from build123d import *

# Parameters (mm, degrees)
SKETCH1_W            = 76
SKETCH1_H            = 16
BOSS_EXTRUDE1_DEPTH  = 1.5
SKETCH2_W            = 6
SKETCH2_H            = 6
BOSS_EXTRUDE2_DEPTH  = 4
SKETCH3_R            = 1.75
BOSS_EXTRUDE3_DEPTH  = 1.5
SKETCH7_W            = 6
SKETCH7_H            = 6
BOSS_EXTRUDE4_DEPTH  = 4
SKETCH9_R            = 1.75
BOSS_EXTRUDE5_DEPTH  = 1.5
SKETCH11_W           = 6
SKETCH11_H           = 6
BOSS_EXTRUDE6_DEPTH  = 4
SKETCH13_R           = 1.75
BOSS_EXTRUDE7_DEPTH  = 1.5
SKETCH15_W           = 6
SKETCH15_H           = 6
BOSS_EXTRUDE8_DEPTH  = 4
SKETCH17_R           = 1.75
BOSS_EXTRUDE9_DEPTH  = 1.5
SKETCH19_W           = 6
SKETCH19_H           = 6
BOSS_EXTRUDE10_DEPTH = 4
SKETCH21_R           = 1.75
BOSS_EXTRUDE11_DEPTH = 1.5
SKETCH23_R           = 1.5
BOSS_EXTRUDE12_DEPTH = 7
FILLET1_R            = 1
SKETCH24_W           = 18
SKETCH24_H           = 9
BOSS_EXTRUDE13_DEPTH = 5
M3_CLEARANCE_HOLE2_D = 3.4


with BuildPart() as part:
    # Sketch1 → Boss-Extrude1 (new body)
    with BuildSketch(Plane.XY):
        with Locations((38, 8)):
            Rectangle(SKETCH1_W, SKETCH1_H)
    extrude(amount=BOSS_EXTRUDE1_DEPTH)

    # Sketch2 → Boss-Extrude2 (add)
    with BuildSketch(Plane.XY.offset(1.5)):
        with Locations((6, 5)):
            Rectangle(SKETCH2_W, SKETCH2_H)
    extrude(amount=BOSS_EXTRUDE2_DEPTH)

    # Sketch3 → Boss-Extrude3 (add)
    with BuildSketch(Plane.XY.offset(5.5)):
        with Locations(Location((6.17, 5, 0), (0, 0, 180))):
            Circle(SKETCH3_R)
    extrude(amount=BOSS_EXTRUDE3_DEPTH)

    # Sketch7 → Boss-Extrude4 (add)
    with BuildSketch(Plane(origin=(16.242371321, -0.520498802, 1.5), x_dir=(1, 0, 0), z_dir=(0, 0, 1))):
        with Locations((7.477628679, 5.520498802)):
            Rectangle(SKETCH7_W, SKETCH7_H)
    extrude(amount=BOSS_EXTRUDE4_DEPTH)

    # Sketch9 → Boss-Extrude5 (add)
    with BuildSketch(Plane(origin=(16.242371321, -0.520498802, 5.5), x_dir=(1, 0, 0), z_dir=(0, 0, 1))):
        with Locations(Location((7.477628679, 5.520498802, 0), (0, 0, 180))):
            Circle(SKETCH9_R)
    extrude(amount=BOSS_EXTRUDE5_DEPTH)

    # Sketch11 → Boss-Extrude6 (add)
    with BuildSketch(Plane(origin=(28.595266875, 2.580968484, 1.5), x_dir=(1, 0, 0), z_dir=(0, 0, 1))):
        with Locations((7.724733125, 2.419031516)):
            Rectangle(SKETCH11_W, SKETCH11_H)
    extrude(amount=BOSS_EXTRUDE6_DEPTH)

    # Sketch13 → Boss-Extrude7 (add)
    with BuildSketch(Plane(origin=(28.595266875, 2.580968484, 5.5), x_dir=(1, 0, 0), z_dir=(0, 0, 1))):
        with Locations(Location((7.724733125, 2.419031516, 0), (0, 0, 180))):
            Circle(SKETCH13_R)
    extrude(amount=BOSS_EXTRUDE7_DEPTH)

    # Sketch15 → Boss-Extrude8 (add)
    with BuildSketch(Plane(origin=(42.206058337, 2.089594669, 1.5), x_dir=(1, 0, 0), z_dir=(0, 0, 1))):
        with Locations((9.813941663, 2.910405331)):
            Rectangle(SKETCH15_W, SKETCH15_H)
    extrude(amount=BOSS_EXTRUDE8_DEPTH)

    # Sketch17 → Boss-Extrude9 (add)
    with BuildSketch(Plane(origin=(42.206058337, 2.089594669, 5.5), x_dir=(1, 0, 0), z_dir=(0, 0, 1))):
        with Locations(Location((9.813941663, 2.910405331, 0), (0, 0, 180))):
            Circle(SKETCH17_R)
    extrude(amount=BOSS_EXTRUDE9_DEPTH)

    # Sketch19 → Boss-Extrude10 (add)
    with BuildSketch(Plane(origin=(52.604179533, 1.086479777, 1.5), x_dir=(1, 0, 0), z_dir=(0, 0, 1))):
        with Locations((17.295820467, 3.913520223)):
            Rectangle(SKETCH19_W, SKETCH19_H)
    extrude(amount=BOSS_EXTRUDE10_DEPTH)

    # Sketch21 → Boss-Extrude11 (add)
    with BuildSketch(Plane(origin=(52.604179533, 1.086479777, 5.5), x_dir=(1, 0, 0), z_dir=(0, 0, 1))):
        with Locations(Location((17.295820467, 3.913520223, 0), (0, 0, 180))):
            Circle(SKETCH21_R)
    extrude(amount=BOSS_EXTRUDE11_DEPTH)

    # Sketch23 → Boss-Extrude12 (add)
    with BuildSketch(Plane.XY.offset(1.5)):
        with Locations(Location((6.17, 10.5, 0), (0, 0, 180))):
            Circle(SKETCH23_R)
    extrude(amount=BOSS_EXTRUDE12_DEPTH)

    # Fillet1
    fillet1_edges = [part.edges().sort_by_distance(p)[0] for p in [
        (7.67, 10.5, 8.5),
    ]]
    fillet(fillet1_edges, radius=FILLET1_R)

    # Sketch24 → Boss-Extrude13 (add)
    with BuildSketch(Plane.XY.offset(1.5)):
        with Locations((38, 17.5)):
            Rectangle(SKETCH24_W, SKETCH24_H)
    extrude(amount=BOSS_EXTRUDE13_DEPTH)

    # M3 Clearance Hole2 (through all)
    with Locations(Plane.XY.offset(1.5)):
        with Locations((16, 5), (60.9, 5)):
            Hole(M3_CLEARANCE_HOLE2_D / 2)


solid = part.part
Geometry check sheet. Reference: the model listing, model coordinates, mm. A direction names the side the tool comes from. Give positions to 0.01 mm unless a question says otherwise; leave off trailing zeros. Loops run counter-clockwise (first coordinate to the right, second up) from the corner with the lowest first, then second, coordinate; pieces in that order, holes last.
(1) Section check C-C on x = 52.02. Record the cut outline in (y, z), then the cut area to 4 significant figures.
From the geometry:
outline: (0, 0) - (16, 0) - (16, 1.5) - (8, 1.5) - (8, 5.5) - (6.75, 5.5) - (6.75, 7) - (3.25, 7) - (3.25, 5.5) - (2, 5.5) - (2, 1.5) - (0, 1.5) - close
area: 53.25 mm2
(2) Thickness scan on L1, parallel to X at y = 7.25, z = 3.75; L2, parallel to Y at x = 16, z = 1.15; L3, parallel to Z at x = 40, y = 14. Record the ranges inside material, lowest first.
From the geometry:
L1: x = 3 to 9, 20.72 to 26.72, 33.32 to 39.32, 49.02 to 55.02, 66.9 to 72.9
L2: y = 0 to 3.3, 6.7 to 16
L3: z = 0 to 6.5
(3) Release check for a two-part mould opening along X. For faces 6 (the flat face through (66.9, 5, 3)), 7 (the flat face through (0, 8, 1)), 8 (the flat face through (52, 5, 7)) record: released by +X, released by -X, zero draft, split by the parting line, or undercut.
From the geometry:
face 6: undercut
face 7: released by -X
face 8: zero draft
(4) Depth check by flat-ended pin: pin 1 Ø2 at (x, z) = (7.5, 3.5) entering from -Y; pin 2 Ø2 at (y, z) = (2.5, 5.5) entering from +X; pin 3 Ø1 at (x, y) = (70, 5) entering from +Z; pin 4 Ø4 at (x, z) = (61.5, 5) entering from +Y. Enter the tip coordinate at first touch or a pass-through.
From the geometry:
pin 1: stops at y = 2
pin 2: stops at x = 72.9
pin 3: stops at z = 7
pin 4: passes through
(5) Section check B-B on z = 2.5. Record the cut outline in (x, y), then the cut area to 3 significant figures.
From the geometry:
outline: (3, 2) - (9, 2) - (9, 8) - (3, 8) - close; circle Ø3 at (6.17, 10.5); (20.72, 2) - (26.72, 2) - (26.72, 8) - (20.72, 8) - close; (29, 13) - (47, 13) - (47, 22) - (29, 22) - close; (33.32, 2) - (39.32, 2) - (39.32, 8) - (33.32, 8) - close; (49.02, 2) - (55.02, 2) - (55.02, 8) - (49.02, 8) - close; (66.9, 2) - (72.9, 2) - (72.9, 8) - (66.9, 8) - close
area: 349 mm2
(6) Section check D-D on y = 17.25. Record the cut outline in (x, z).
From the geometry:
outline: (29, 1.5) - (47, 1.5) - (47, 6.5) - (29, 6.5) - close
(7) Set-up check for faces 1 (the flat face through (36, 8, 3)), 2 (the flat face through (24, 8, 3)), 3 (the flat face through (3, 5, 3)), 4 (the flat face through (52, 2, 3)), 5 (the cylindrical face through (50.403, 5.67, 6.24)): record each of +Z, -Z, +X, -X, +Y, -Y from which the full face is reachable in a straight line by a thin tool's end or side.
From the geometry:
face 1: +Z, +X, -X
face 2: +Z, +X, -X, +Y
face 3: +Z, -X, +Y, -Y
face 4: +Z, +X, -X, -Y
face 5: +Z
(8) Section check A-A on x = 16. Record the cut outline in (y, z).
From the geometry:
outline: (0, 0) - (3.3, 0) - (3.3, 1.5) - (0, 1.5) - close; (6.7, 0) - (16, 0) - (16, 1.5) - (6.7, 1.5) - close
